```python
from build123d import *
from build123d.topology import SkipClean

# Parameters (mm, degrees)
SALIENTE_EXTRUIR1_DEPTH = 5
CROQUIS2_R              = 2.1
CORTAR_EXTRUIR1_DEPTH   = 83.176639016
CORTAR_EXTRUIR2_DEPTH   = 83.176639016
CROQUIS5_R              = 2.05
CORTAR_EXTRUIR4_DEPTH   = 83.176639016
SALIENTE_EXTRUIR2_DEPTH = 5
CORTAR_EXTRUIR10_DEPTH  = 98.128780493
SALIENTE_EXTRUIR4_DEPTH = 4
SALIENTE_EXTRUIR5_DEPTH = 4
CROQUIS17_R             = 2.4
CORTAR_EXTRUIR11_DEPTH  = 98.128780493


with BuildPart() as part:
    # Croquis1 → Saliente-Extruir1 (new body)
    with BuildSketch(Plane(origin=(0, 0, 0), x_dir=(1, 0, 0), z_dir=(0, 1, 0))):
        with BuildLine():
            Line((4, 58), (8.807070745, 49.218243619))
            ThreePointArc((8.807070745, 49.218243619), (35.355339059, 35.355339059), (49.218243619, 8.807070745))
            Line((49.218243619, 8.807070745), (58, 4))
            Line((58, 4), (58, -4))
            Line((58, -4), (49.218243619, -8.807070745))
            ThreePointArc((49.218243619, -8.807070745), (35.355339059, -35.355339059), (8.807070745, -49.218243619))
            Line((8.807070745, -49.218243619), (4, -58))
            Line((4, -58), (-4, -58))
            Line((-4, -58), (-8.807070745, -49.218243619))
            ThreePointArc((-8.807070745, -49.218243619), (-35.355339059, -35.355339059), (-49.218243619, -8.807070745))
            Line((-49.218243619, -8.807070745), (-58, -4))
            Line((-58, -4), (-58, 4))
            Line((-58, 4), (-49.218243619, 8.807070745))
            ThreePointArc((-49.218243619, 8.807070745), (-35.355339059, 35.355339059), (-8.807070745, 49.218243619))
            Line((-8.807070745, 49.218243619), (-4, 58))
            Line((-4, 58), (4, 58))
        make_face()
    extrude(amount=SALIENTE_EXTRUIR1_DEPTH)

    # Croquis2 → Cortar-Extruir1 (cut, through all)
    with BuildSketch(Plane(origin=(0, 5, 0), x_dir=(1, 0, 0), z_dir=(0, 1, 0))):
        with Locations(Location((0, 52.7, 0), (0, 0, 270))):
            Circle(CROQUIS2_R)
        with Locations(Location((52.7, 0, 0), (0, 0, 270))):
            Circle(CROQUIS2_R)
        with Locations(Location((0, -52.7, 0), (0, 0, 270))):
            Circle(CROQUIS2_R)
        with Locations(Location((-52.7, 0, 0), (0, 0, 270))):
            Circle(CROQUIS2_R)
    extrude(amount=-CORTAR_EXTRUIR1_DEPTH, mode=Mode.SUBTRACT)

    # Croquis3 → Cortar-Extruir2 (cut, through all)
    with BuildSketch(Plane(origin=(0, 5, 0), x_dir=(1, 0, 0), z_dir=(0, 1, 0))):
        Polygon((20.506096654, -34.648232278), (34.648232278, -20.506096654), (47.376154339, -33.234018716), (67.218949341, -53.076813717), (53.076813717, -67.218949341), (33.234018716, -47.376154339), align=None)
    extrude(amount=-CORTAR_EXTRUIR2_DEPTH, mode=Mode.SUBTRACT)

    # Croquis5 → Cortar-Extruir4 (cut, through all)
    with BuildSketch(Plane(origin=(0, 5, 0), x_dir=(1, 0, 0), z_dir=(0, 1, 0))):
        with Locations(Location((-7.78, 7.78, 0), (0, 0, 270))):
            Circle(CROQUIS5_R)
        with Locations(Location((7.78, 7.78, 0), (0, 0, 270))):
            Circle(CROQUIS5_R)
        with Locations(Location((7.78, -7.78, 0), (0, 0, 270))):
            Circle(CROQUIS5_R)
        with Locations(Location((-7.78, -7.78, 0), (0, 0, 270))):
            Circle(CROQUIS5_R)
        with BuildLine():
            Line((21.554064831, -30.039346205), (23.334523779, -31.819805153))
            Line((23.334523779, -31.819805153), (24.748737342, -30.405591591))
            Line((24.748737342, -30.405591591), (22.968278393, -28.625132642))
            ThreePointArc((22.968278393, -28.625132642), (19.622213178, -26.69328099), (21.554064831, -30.039346205))
        make_face()
        with BuildLine():
            Line((28.625132642, -22.968278393), (30.986174209, -25.329319959))
            Line((30.986174209, -25.329319959), (32.400387771, -23.915106397))
            Line((32.400387771, -23.915106397), (30.039346205, -21.554064831))
            ThreePointArc((30.039346205, -21.554064831), (26.69328099, -19.622213178), (28.625132642, -22.968278393))
        make_face()
    extrude(amount=-CORTAR_EXTRUIR4_DEPTH, mode=Mode.SUBTRACT)

    # Croquis7 → Saliente-Extruir2 (add, through all)
    with BuildSketch(Plane(origin=(0, 5, 0), x_dir=(1, 0, 0), z_dir=(0, 1, 0))):
        Polygon((68.589357775, -54.447222151), (54.447222151, -68.589357775), (8.807070745, -49.218243619), (18.571685103, -46.422973972), (27.56994834, -41.712083963), (48.790367902, -62.932503526), (62.932503526, -48.790367902), (41.712083963, -27.56994834), (46.422973972, -18.571685103), (49.218243619, -8.807070745), align=None)
    extrude(amount=-SALIENTE_EXTRUIR2_DEPTH)

    # Croquis8 → Cortar-Extruir10 (cut, through all)
    with BuildSketch(Plane(origin=(0, 5, 0), x_dir=(1, 0, 0), z_dir=(0, 1, 0))):
        with BuildLine():
            Line((54.283137452, -59.939991701), (51.490214314, -57.147068564))
            Line((51.490214314, -57.147068564), (50.076000752, -58.561282126))
            Line((50.076000752, -58.561282126), (52.868923889, -61.354205264))
            ThreePointArc((52.868923889, -61.354205264), (56.214989104, -63.286056916), (54.283137452, -59.939991701))
        make_face()
        with BuildLine():
            Line((57.371843354, -51.714989104), (58.786056916, -50.300775542))
            Line((58.786056916, -50.300775542), (61.354205264, -52.868923889))
            ThreePointArc((61.354205264, -52.868923889), (63.286056916, -56.214989104), (59.939991701, -54.283137452))
            Line((59.939991701, -54.283137452), (57.371843354, -51.714989104))
        make_face()
    extrude(amount=-CORTAR_EXTRUIR10_DEPTH, mode=Mode.SUBTRACT)

    # Croquis15 → Saliente-Extruir4 (add)
    with BuildSketch(Plane.XZ):
        with BuildLine():
            Line((-1.111111111, -20.469866441), (-1.111111111, -22.472548411))
            ThreePointArc((-1.111111111, -22.472548411), (0, 22.5), (1.111111111, -22.472548411))
            Line((1.111111111, -22.472548411), (1.111111111, -20.469866441))
            ThreePointArc((1.111111111, -20.469866441), (0, 20.5), (-1.111111111, -20.469866441))
        make_face()
    extrude(amount=SALIENTE_EXTRUIR4_DEPTH)

    # Croquis16 → Saliente-Extruir5 (add)
    with SkipClean():  # the faces are left unmerged after this step: merging them gives an invalid solid
        with BuildSketch(Plane.XZ):
            with BuildLine():
                Line((-1.111111111, -20.469866441), (-1.111111111, -22.472548411))
                ThreePointArc((-1.111111111, -22.472548411), (0, -22.5), (1.111111111, -22.472548411))
                Line((1.111111111, -22.472548411), (1.111111111, -20.469866441))
                ThreePointArc((1.111111111, -20.469866441), (0, -20.5), (-1.111111111, -20.469866441))
            make_face()
        extrude(amount=SALIENTE_EXTRUIR5_DEPTH)

    # Croquis17 → Cortar-Extruir11 (cut, through all)
    with SkipClean():  # the faces are left unmerged after this step: merging them gives an invalid solid
        with BuildSketch(Plane.XZ):
            with Locations(Location((42.43, 0, 0), (0, 0, 270))):
                Circle(CROQUIS17_R)
            with Locations(Location((0, -42.43, 0), (0, 0, 270))):
                Circle(CROQUIS17_R)
            with Locations(Location((-42.43, 0, 0), (0, 0, 270))):
                Circle(CROQUIS17_R)
            with Locations(Location((0, 42.43, 0), (0, 0, 270))):
                Circle(CROQUIS17_R)
        extrude(amount=-CORTAR_EXTRUIR11_DEPTH, mode=Mode.SUBTRACT)


solid = part.part
```
Geometry: final body of the model. Coordinates: model frame, mm. A direction names the side the tool comes from. Coordinates: 2 decimals unless noted, no trailing zeros. Order: outer loops, then holes, each group sorted by start corner. A loop starts at its lowest first (then second) coordinate and runs counter-clockwise, first axis right, second up. Notation, with made-up numbers: M 16,16.25 L 37,16.25 A4 ccw 37,20.25 Z; hole C -17,-18 d9. An arc over 180 degrees is marked long. Answer in a Markdown table with one row per item. Add a question column.
Q1. Contact query for flat-ended pins moving along their axis: P1, Ø20.5, axis at x = -9, z = -3.5, coming from the -Y side; P2, Ø1.5, axis at x = -2, y = 1.5, coming from the +Z side; P3, Ø1, axis at x = -14, y = -1, coming from the -Z side. Output: stop coordinate, or through.
Q2. Section query D-D on z = -42.43. Return the cut outline in (x, y), and give its area (3 significant figures).
Q3. Line query: L1, parallel to X at y = 2.1, z = 0; L2, parallel to Z at x = 7, y = 2; L3, parallel to Z at x = 57, y = 0.5. Output: solid intervals per line, ascending.
Q4. Section query A-A on z = 0. Return the cut outline in (x, y).
Q5. Reachability of faces 1 (the flat face through (31.95, 2.54, 59.04)), 2 (the flat face through (0, 0, 0)), 3 (the flat face through (58.77, 2.54, 31.31)), 4 (the flat face through (50.185, 2.535, 61.538)), 5 (the flat face through (0, 2, 58)) from +Z, -Z, +X, -X, +Y, -Y: full face, straight path, thin tool, end or side. Return the list, or none.
Q6. Section query C-C on y = 2.5. Count the separate pieces of the cut face and the enclosed holes in it, and give its area (3 significant figures).
Q7. Section query B-B on x = -52.7. Return the cut outline in (y, z).
Q8. Mould query, pull axis Z, two halves, no side actions, for faces 6 (the flat face through (53.548, 2.465, -6.437)), 7 (the flat face through (18.2, -4, -9.9)), 8 (the cylindrical face through (6.533, 2.535, -9.407)). Classes: released by +Z, released by -Z, zero draft, split by the parting line, or undercut.
Completed:
| question | item | result |
|---|---|---|
| 1 | P1 | stops at y = 0 |
| 1 | P2 | stops at z = 58 |
| 1 | P3 | stops at z = -18 |
| 2 | outline | M -26.45,0 L -2.4,0 L -2.4,5 L -26.45,5 Z; M 2.4,0 L 26.45,0 L 26.45,5 L 2.4,5 Z |
| 2 | area | 241 mm2 |
| 3 | L1 | x = -58 to -54.8, -50.6 to -44.83, -40.03 to 40.03, 44.83 to 50.6, 54.8 to 58 |
| 3 | L2 | z = -52.52 to -9.68, -5.88 to 5.88, 9.68 to 52.52 |
| 3 | L3 | z = -4.55 to 4.55, 27.14 to 42.86, 54.72 to 66.04 |
| 4 | outline | M -58,0 L -54.8,0 L -54.8,5 L -58,5 Z; M -50.6,0 L -44.83,0 L -44.83,5 L -50.6,5 Z; M -40.03,0 L -22.5,0 L -22.5,-4 L -20.5,-4 L -20.5,0 L 20.5,0 L 20.5,-4 L 22.5,-4 L 22.5,0 L 40.03,0 L 40.03,5 L -40.03,5 Z; M 44.83,0 L 50.6,0 L 50.6,5 L 44.83,5 Z; M 54.8,0 L 58,0 L 58,5 L 54.8,5 Z |
| 5 | face 1 | +Z, +Y, -Y |
| 5 | face 2 | -Y |
| 5 | face 3 | +X, +Y, -Y |
| 5 | face 4 | +Y, -Y |
| 5 | face 5 | +Z, -X, +Y, -Y |
| 6 | separate pieces | 1 |
| 6 | enclosed holes | 13 |
| 6 | area | 8,650 mm2 |
| 7 | outline | M 0,-6.9 L 5,-6.9 L 5,-2.1 L 0,-2.1 Z; M 0,2.1 L 5,2.1 L 5,6.9 L 0,6.9 Z |
| 8 | face 6 | released by -Z |
| 8 | face 7 | zero draft |
| 8 | face 8 | undercut |
